Input: part model. Units: mm. Frame: model coordinates. Face numbers are marked on the shaded views. Coordinates: 2 decimals unless noted, no trailing zeros. Order: outer loops, then holes, each group sorted by start corner. A loop starts at its lowest first (then second) coordinate and runs counter-clockwise, first axis right, second up.
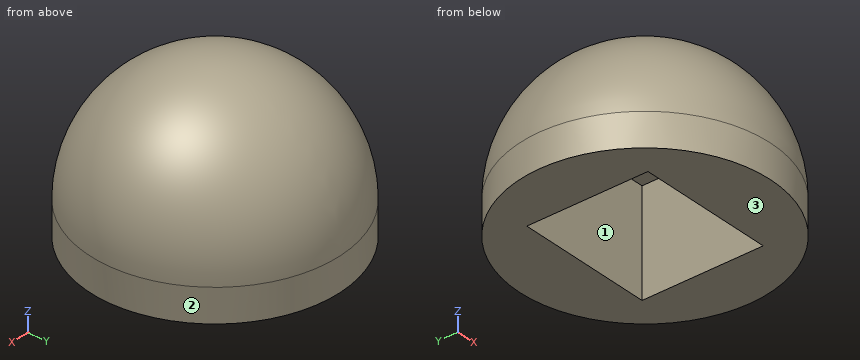
from build123d import *

# Parameters (mm, degrees)
SKIZZE3_W                       = 3.3
SKIZZE3_H                       = 2.9
SCHNITT_LINEAR_AUSTRAGEN1_DEPTH = 2.5


with BuildPart() as part:
    # Skizze2 → Rotation2 (revolve)
    with BuildSketch(Plane(origin=(0, 0, 0), x_dir=(0, 0, -1), z_dir=(1, 0, 0))):
        with BuildLine():
            Line((-0.8, 3), (0, 3))
            Line((0, 3), (0, 0))
            Line((0, 0), (-3.8, 0))
            ThreePointArc((-3.8, 0), (-2.921320344, 2.121320344), (-0.8, 3))
        make_face()
    revolve(axis=Axis((0, 0, 0.8), (0, 0, 1)))

    # Skizze3 → Schnitt-Linear austragen1 (cut)
    with BuildSketch(Plane(origin=(0, 0, 0), x_dir=(-1, 0, 0), z_dir=(0, 0, -1))):
        Rectangle(SKIZZE3_W, SKIZZE3_H)
    extrude(amount=-SCHNITT_LINEAR_AUSTRAGEN1_DEPTH, mode=Mode.SUBTRACT)


solid = part.part
Item 1: Pin query (flat end, axial travel): pin 1 Ø1.5 at (x, y) = (2.5, -2) entering from +Z; pin 2 Ø0.8 at (y, z) = (0.5, 1.5) entering from +X; pin 3 Ø1.2 at (y, z) = (-0.5, 1.5) entering from -X. Return the tip coordinate at first contact, or that it passes through.
Response values:
pin 1: stops at z = 2.53
pin 2: stops at x = 2.96
pin 3: stops at x = -2.99
Item 2: Cut plane A-A on y = 0. Return loops of the section in (x, z).
Response values:
outline: (-3, 0) - (-1.65, 0) - (-1.65, 2.5) - (1.65, 2.5) - (1.65, 0) - (3, 0) - (3, 0.8) arc R3 ccw to (-3, 0.8) - close
Item 3: Draft query along X for the marked faces 1, 2 and 3. Return one class per face: pulls with the +X half, pulls with the -X half, needs draft (parallel to the pull), parting line crosses it, or undercut.
Response values:
face 1: undercut
face 2: parting line crosses it
face 3: needs draft
Item 4: Cut plane B-B on z = 0.5. Return loops of the section in (x, y).
Response values:
outline: circle Ø6 at (0, 0); hole (-1.65, -1.45) - (1.65, -1.45) - (1.65, 1.45) - (-1.65, 1.45) - close
Item 5: Cut plane C-C on x = 0. Return loops of the section in (y, z), then the cut area to 3 significant figures.
Response values:
outline: (-3, 0) - (-1.45, 0) - (-1.45, 2.5) - (1.45, 2.5) - (1.45, 0) - (3, 0) - (3, 0.8) arc R3 ccw to (-3, 0.8) - close
area: 11.7 mm2
Item 6: Ray query, probe 1 along X at (y, z) = (-0.7, 2.1); probe 2 along Z at (x, y) = (-0.05, 0.1); probe 3 along Y at (x, z) = (1.5, 1.3). Return the intervals inside material, ascending.
Response values:
probe 1: x = -2.61 to -1.65, 1.65 to 2.61
probe 2: z = 2.5 to 3.8
probe 3: y = -2.55 to -1.45, 1.45 to 2.55
Item 7: Cut plane D-D on y = -1. Return loops of the section in (x, z), then the cut area to 3 significant figures.
Response values:
outline: (-2.83, 0) - (-1.65, 0) - (-1.65, 2.5) - (1.65, 2.5) - (1.65, 0) - (2.83, 0) - (2.83, 0.8) arc R2.83 ccw to (-2.83, 0.8) - close
area: 8.84 mm2
